Geometry: final body of the model. Coordinates: model frame, mm. A direction names the side the tool comes from. Round coordinates to 2 decimals unless told otherwise and drop trailing zeros. Loops run counter-clockwise (first coordinate to the right, second up) from the corner with the lowest first, then second, coordinate; pieces in that order, holes last. Notation, with made-up numbers: M 16.25,11 L 38.25,11 A24 ccw 38.25,39 Z; hole C 23,-11.75 d1. An arc over 180 degrees is marked long. Answer as a JSON object with one key per item and string values.
from build123d import *

# Parameters (mm, degrees)
SKETCH_W        = 55
SKETCH_H        = 60
PAD_DEPTH       = 14
SKETCH001_R     = 7.6
POCKET_DEPTH    = 60.001
SKETCH002_R     = 1.75
POCKET001_DEPTH = 14.001
POCKET002_DEPTH = 12
SKETCH004_R     = 2.25
POCKET003_DEPTH = 14.001
SKETCH008_R     = 4.1
POCKET005_DEPTH = 20
SKETCH010_W     = 20
SKETCH010_H     = 25
POCKET006_DEPTH = 5
SKETCH011_R     = 2.25
POCKET007_DEPTH = 10
CHAMFER_SIZE    = 3
CHAMFER001_SIZE = 3
POCKET008_DEPTH = 4.5


with BuildPart() as part:
    # Sketch → Pad (new body)
    with BuildSketch(Plane.XY):
        with Locations((17.5, 0)):
            Rectangle(SKETCH_W, SKETCH_H)
    extrude(amount=PAD_DEPTH)

    # Sketch001 → Pocket (cut, through all)
    with BuildSketch(Plane.XZ.offset(30)):
        with Locations((0, 14)):
            Circle(SKETCH001_R)
    extrude(amount=-POCKET_DEPTH, mode=Mode.SUBTRACT)

    # Sketch002 → Pocket001 (cut, through all)
    with BuildSketch(Plane(origin=(0, 0, 0), x_dir=(1, 0, 0), z_dir=(0, 0, -1))):
        with Locations((-6, 27)):
            Circle(SKETCH002_R)
        with Locations((-6, -27)):
            Circle(SKETCH002_R)
        with Locations((6, 27)):
            Circle(SKETCH002_R)
        with Locations((6, -27)):
            Circle(SKETCH002_R)
        with Locations((6, 0)):
            Circle(SKETCH002_R)
        with Locations((-6, 0)):
            Circle(SKETCH002_R)
    extrude(amount=-POCKET001_DEPTH, mode=Mode.SUBTRACT)

    # Sketch003 → Pocket002 (cut)
    with BuildSketch(Plane.XY.offset(14)):
        with BuildLine():
            Line((10, 35), (10, -35))
            Line((10, -35), (28, -35))
            Line((28, -35), (28, -14.916198))
            ThreePointArc((28, -14.916198), (30.841983, -12.965458), (32.599342, -10))
            Line((32.599342, -10), (52.599342, -10))
            Line((52.599342, -10), (52.599342, 10))
            Line((52.599342, 10), (32.599342, 10))
            ThreePointArc((32.599342, 10), (30.841983, 12.965458), (28, 14.916198))
            Line((28, 14.916198), (28, 35))
            Line((28, 35), (10, 35))
        make_face()
    extrude(amount=-POCKET002_DEPTH, mode=Mode.SUBTRACT)

    # Sketch004 → Pocket003 (cut, through all)
    with BuildSketch(Plane(origin=(0, 0, 0), x_dir=(1, 0, 0), z_dir=(0, 0, -1))):
        with Locations((25, 7.5)):
            Circle(SKETCH004_R)
        with Locations((25, -7.5)):
            Circle(SKETCH004_R)
    extrude(amount=-POCKET003_DEPTH, mode=Mode.SUBTRACT)

    # Sketch008 → Pocket005 (cut)
    with BuildSketch(Plane.YZ.offset(45)):
        with Locations((-20, 14)):
            Circle(SKETCH008_R)
        with Locations((20, 14)):
            Circle(SKETCH008_R)
    extrude(amount=-POCKET005_DEPTH, mode=Mode.SUBTRACT)

    # Sketch010 → Pocket006 (cut)
    with BuildSketch(Plane.YZ.offset(45)):
        with Locations((0, 6.5)):
            Rectangle(SKETCH010_W, SKETCH010_H)
    extrude(amount=-POCKET006_DEPTH, mode=Mode.SUBTRACT)

    # Sketch011 → Pocket007 (cut)
    with BuildSketch(Plane.XY.offset(14)):
        with Locations((36, 27)):
            Circle(SKETCH011_R)
        with Locations((36, 13)):
            Circle(SKETCH011_R)
        with Locations((36, -13)):
            Circle(SKETCH011_R)
        with Locations((36, -27)):
            Circle(SKETCH011_R)
    extrude(amount=-POCKET007_DEPTH, mode=Mode.SUBTRACT)

    # Chamfer
    chamfer_edges = [part.edges().sort_by_distance(p)[0] for p in [
        (45, -10, 8),
        (45, -10, 1),
    ]]
    chamfer(chamfer_edges, length=CHAMFER_SIZE)

    # Chamfer001
    chamfer001_edges = [part.edges().sort_by_distance(p)[0] for p in [
        (45, 10, 8),
        (45, 10, 1),
    ]]
    chamfer(chamfer001_edges, length=CHAMFER001_SIZE)

    # Sketch012 → Pocket008 (cut)
    with BuildSketch(Plane(origin=(0, 0, 0), x_dir=(1, 0, 0), z_dir=(0, 0, -1))):
        Polygon((-4.412285, 29.750003), (-7.587715, 29.750003), (-9.17543, 27), (-7.587715, 24.249997), (-4.412285, 24.249997), (-2.82457, 27), align=None)
        Polygon((7.587715, 29.750003), (4.412285, 29.750003), (2.82457, 27), (4.412285, 24.249997), (7.587715, 24.249997), (9.17543, 27), align=None)
        Polygon((-4.412285, 2.750003), (-7.587715, 2.750003), (-9.17543, 0), (-7.587715, -2.750003), (-4.412285, -2.750003), (-2.82457, 0), align=None)
        Polygon((7.587715, 2.750003), (4.412285, 2.750003), (2.82457, 0), (4.412285, -2.750003), (7.587715, -2.750003), (9.17543, 0), align=None)
        Polygon((-4.412285, -24.249997), (-7.587715, -24.249997), (-9.17543, -27), (-7.587715, -29.750003), (-4.412285, -29.750003), (-2.82457, -27), align=None)
        Polygon((7.587715, -24.249997), (4.412285, -24.249997), (2.82457, -27), (4.412285, -29.750003), (7.587715, -29.750003), (9.17543, -27), align=None)
    extrude(amount=-POCKET008_DEPTH, mode=Mode.SUBTRACT)


solid = part.part
1) Section query D-D (y = 20). Return the cut outline in (x, z), and give its area (3 significant figures).
Results:
{"outline": "M -10,0 L 45,0 L 45,9.9 L 28,9.9 L 28,2 L 10,2 L 10,14 L 7.6,14 A7.6 cw -7.6,14 L -10,14 Z", "area": "394 mm2"}
2) Pull-direction query (X, two-part tool) for faces 4 (the flat face through (3.61, -25.64, 2.22)), 5 (the flat face through (23, -30, 1)), 6 (the flat face through (45, 21, 7)); classes: +X half, -X half, draft (parallel to the pull), parting line (faces both ways), or undercut.
Results:
{"face 4": "undercut", "face 5": "draft", "face 6": "+X half"}
3) Section query A-A (x = 25). Return the cut outline in (y, z), and give its area (3 significant figures).
Results:
{"outline": "M -30,0 L -9.75,0 L -9.75,2 L -30,2 Z; M -5.25,0 L 5.25,0 L 5.25,2 L -5.25,2 Z; M 9.75,0 L 30,0 L 30,2 L 9.75,2 Z", "area": "102 mm2"}
4) Pin query (flat end, axial travel): P1, Ø5, axis at x = -1.5, y = 14, coming from the +Z side; P2, Ø3, axis at x = 19, y = 18, coming from the +Z side; P3, Ø3.5, axis at y = 0, z = 10, coming from the +X side. Return the tip coordinate at first contact, or that it passes through.
Results:
{"P1": "z = 7.54", "P2": "z = 2", "P3": "x = 10"}
5) Section query C-C (z = 9). Count the separate pieces of the cut face and the enclosed holes in it, and give its area (3 significant figures).
Results:
{"separate pieces": "4", "enclosed holes": "4", "area": "1,060 mm2"}
6) Reachability of faces 1 (the cylindrical face through (27.146, 6.824, 0.986)), 2 (the flat face through (-6, -2.75, 2)), 3 (the flat face through (36, 27, 4)) from +Z, -Z, +X, -X, +Y, -Y: full face, straight path, thin tool, end or side. Return the list, or none.
Results:
{"face 1": "+Z, -Z", "face 2": "-Z", "face 3": "+Z"}
7) Ray query, line 1 (Y direction, x = 25, z = 1.35); line 2 (Y direction, x = -5, z = 2.5); line 3 (Y direction, x = 6, z = 7). Return the intervals inside material, ascending.
Results:
{"line 1": "-30 to -9.75, -5.25 to 5.25, 9.75 to 30", "line 2": "-30 to -29.75, -24.25 to -2.75, 2.75 to 24.25, 29.75 to 30", "line 3": "-30 to -28.75, -25.25 to -1.75, 1.75 to 25.25, 28.75 to 30"}
8) Section query B-B (x = 6). Return the cut outline in (y, z), and give its area (3 significant figures).
Results:
{"outline": "M -30,0 L -29.75,0 L -29.75,4.5 L -28.75,4.5 L -28.75,9.34 L -30,9.34 Z; M -25.25,4.5 L -24.25,4.5 L -24.25,0 L -2.75,0 L -2.75,4.5 L -1.75,4.5 L -1.75,9.34 L -25.25,9.34 Z; M 1.75,4.5 L 2.75,4.5 L 2.75,0 L 24.25,0 L 24.25,4.5 L 25.25,4.5 L 25.25,9.34 L 1.75,9.34 Z; M 28.75,4.5 L 29.75,4.5 L 29.75,0 L 30,0 L 30,9.34 L 28.75,9.34 Z", "area": "435 mm2"}
